```python
from build123d import *

# Parameters (mm, degrees)
BOSS_EXTRUDE1_DEPTH     = 15
CUT_EXTRUDE2_DEPTH      = 58
CUT_EXTRUDE2_DEPTH_BACK = 63


with BuildPart() as part:
    # Sketch1 → Boss-Extrude1 (new body)
    with BuildSketch(Plane(origin=(0, 0, 0), x_dir=(1, 0, 0), z_dir=(0, 1, 0))):
        with BuildLine():
            Line((-40, -45), (-40.554700196, -35.015396468))
            Line((-40.554700196, -35.015396468), (-40.751707535, -35.387312812))
            ThreePointArc((-40.751707535, -35.387312812), (-37.497275944, 0.081671518), (-44.445299804, 35.015396468))
            Line((-44.445299804, 35.015396468), (-44.722649902, 40.007698234))
            ThreePointArc((-44.722649902, 40.007698234), (0.805300702, 44.940375619), (45, 32.94228634))
            ThreePointArc((45, 32.94228634), (42.479652573, -6.346996403), (35, -45))
            ThreePointArc((35, -45), (-2.5, -42.500708249), (-40, -45))
        make_face()
    extrude(amount=BOSS_EXTRUDE1_DEPTH)

    # Sketch3 → Cut-Extrude2 (cut, two sides)
    with BuildSketch(Plane.XY) as cut_extrude2_sk:
        with BuildLine():
            Line((-49.722649902, 5), (-49.722649902, -2.927919572))
            Line((-49.722649902, -2.927919572), (50, -2.927919572))
            Line((50, -2.927919572), (50, 5))
            ThreePointArc((50, 5), (0.138675049, 10.0002316), (-49.722649902, 5))
        make_face()
    extrude(amount=CUT_EXTRUDE2_DEPTH, mode=Mode.SUBTRACT)
    extrude(cut_extrude2_sk.sketch, amount=-CUT_EXTRUDE2_DEPTH_BACK, mode=Mode.SUBTRACT)


solid = part.part
```
Build history of the part. All positions in model axes, mm. Give positions to 0.01 mm unless a question says otherwise; leave off trailing zeros. Loops run counter-clockwise (first coordinate to the right, second up) from the corner with the lowest first, then second, coordinate; pieces in that order, holes last. Notation, with made-up numbers: (6.5, 15.25) - (60.5, 15.25) arc R18 ccw to (60.5, 47.25) - close; hole circle Ø1 at (10, -36.5). An arc over 180 degrees is marked (long way). Use a Markdown table: item, result.
(1) Drop flat-ended pins along their axis: pin 1 Ø5 at (x, y) = (-21, 11) entering from +Z; pin 2 Ø4 at (x, y) = (-13, 8.5) entering from -Z; pin 3 Ø1 at (y, z) = (8.5, -31.5) entering from -X; pin 4 Ø3 at (x, y) = (-19.5, 7.5) entering from +Z. Give the stop position or say it passes through.
Taken from the geometry:
| item | result |
|---|---|
| pin 1 | z = 43.28 |
| pin 2 | z = -45.3 |
| pin 3 | x = -43.42 |
| pin 4 | through |
(2) Wall check: line 1 along Z through (x, y) = (20.5, 10.75); line 2 along Z through (x, y) = (0, 12.5); line 3 along X through (y, z) = (13.75, 35.5). Give the ranges that are in metal, low to high.
Taken from the geometry:
| item | result |
|---|---|
| line 1 | -41.77 to 43.44 |
| line 2 | -45 to 42.51 |
| line 3 | -40.53 to 37.31 |
(3) Band-saw the part on B-B (x = 22.5). Give the cut face in (y, z), and give its area (3 significant figures).
Taken from the geometry:
| item | result |
|---|---|
| outline | (9, -41.27) - (15, -41.27) - (15, 43.61) - (9, 43.61) - close |
| area | 509 mm2 |
(4) Band-saw the part on A-A (y = 12.75). Give the cut face in (x, z) (1 decimal).
Taken from the geometry:
| item | result |
|---|---|
| outline | (-44.7, -40) arc R123.5 ccw to (45, -32.9) arc R310 ccw to (35, 45) arc R282.6 cw to (-40, 45) - (-40.6, 35) - (-40.8, 35.4) arc R124.2 cw to (-44.4, -35) - close |
(5) Band-saw the part on C-C (z = -7). Give the cut face in (x, y), and give its area (3 significant figures).
Taken from the geometry:
| item | result |
|---|---|
| outline | (-38.05, 7.08) arc R251.1 cw to (43.9, 6.16) - (43.9, 15) - (-38.05, 15) - close |
| area | 503 mm2 |
(6) Pull direction X, two halves, no side cores. Call faces 1 (the face through (1, 15, -1)), 2 (the face through (-44.582, 10.417, -37.477)), 3 (the face through (-2, 11.7, 42.5)): +X half, -X half, draft (parallel to the pull), parting line (faces both ways), or undercut.
Taken from the geometry:
| item | result |
|---|---|
| face 1 | draft |
| face 2 | -X half |
| face 3 | undercut |
